Autodesk Inventor part; units mm, degrees
ref_plane "YZ Plane" through (0, 0, 0) normal (1, 0, 0) x (0, 1, 0)
ref_plane "XZ Plane" through (0, 0, 0) normal (0, 1, 0) x (-1, 0, 0)
ref_plane "XY Plane" through (0, 0, 0) normal (0, 0, 1) x (1, 0, 0)
sketch "Sketch1" plane through (0, 0, 0) normal (0, 1, 0) x (-1, 0, 0)
  line L0 (-33.8, -50.05) -> (33.8, -50.05)
  line L1 (33.8, -50.05) -> (33.8, 50.05)
  line L2 (33.8, 50.05) -> (-33.8, 50.05)
  line L3 (-33.8, 50.05) -> (-33.8, -50.05)
  line L4 (-33.8, -50.05) -> (33.8, 50.05) construction
  line L5 (33.8, -50.05) -> (-33.8, 50.05) construction
  point P0 (0, 0)
  dimension "d0" = 67.6
  dimension "d1" = 100.1
extrude "Extrusion1" add sketch "Sketch1" along normal blind 4.445
sketch "Sketch2" plane through (0, 4.445, 0) normal (0, 1, 0) x (1, 0, 0)
  line L0 (30.6, 46.85) -> (-30.6, 46.85)
  line L1 (-30.6, 46.85) -> (-30.6, -46.85)
  line L2 (-30.6, -46.85) -> (30.6, -46.85)
  line L3 (30.6, -46.85) -> (30.6, 46.85)
  line L4 (30.6, 46.85) -> (-30.6, -46.85) construction
  line L5 (-30.6, 46.85) -> (30.6, -46.85) construction
  line L6 (-33.8, 50.05) -> (-33.8, -50.05)
  line L7 (-33.8, -50.05) -> (33.8, -50.05)
  line L8 (33.8, 50.05) -> (-33.8, 50.05)
  line L9 (33.8, -50.05) -> (33.8, 50.05)
  line L10 (27.4, -43.65) -> (33.8, -50.05) construction
  line L11 (24.9431, -46.85) -> (30.9716, -52.8784)
  line L12 (36.6284, -47.2216) -> (30.6, -41.1931)
  arc A0 (30.9716, -52.8784) -> (36.6284, -47.2216) centre (33.8, -50.05) ccw
  circle A1 centre (33.8, -50.05) radius 1.375
  point P0 (0, 0)
  dimension "d4" = 3.2
  dimension "d5" = 3.2
  dimension "d22" = 8
  dimension "d23" = 2.75
extrude "Extrusion2" add sketch "Sketch2" along normal blind 28 contours L0 L1 L2 L11 L7 L6 L8 L9 L12 L3 | L12 L9 A1 L7 L11 L2 L3 | L9 L7 A1 picked at (32.9402, -49.7491)
sketch "Sketch4" plane through (0, 0, 0) normal (0, -1, 0) x (1, 0, 0)
  line L0 (32.2906, 48.7379) -> (35.3094, 51.3621) construction
  line L1 (33.8, 50.05) -> (33.8, -50.05)
  line L2 (33.8, 44.7499) -> (37.9337, 48.3433)
  line L3 (32.6852, 54.381) -> (29.6663, 51.7567)
  arc A0 (29.6663, 51.7567) -> (28.5119, 50.05) centre (32.2906, 48.7379) ccw
  arc A1 (37.9337, 48.3433) -> (32.6852, 54.381) centre (35.3094, 51.3621) ccw
  line L4 (-33.8, 50.05) -> (33.8, 50.05)
  line L5 (28.5119, 50.05) -> (33.8, 50.05)
  line L6 (33.8, 50.05) -> (33.8, 44.7499)
  circle A2 centre (35.3094, 51.3621) radius 1.985
  line L7 (0, 50.05) -> (0, -50.05) construction
  line L8 (33.8, -50.05) -> (-33.8, -50.05) construction
  line L9 (33.8, 0) -> (-33.3, 0) construction
  line L10 (33.8, -50.05) -> (33.8, 50.05)
  line L11 (33.8, -44.7499) -> (37.9337, -48.3433)
  line L12 (32.6852, -54.381) -> (29.6663, -51.7567)
  arc A3 (28.5119, -50.05) -> (29.6663, -51.7567) centre (32.2906, -48.7379) ccw
  arc A4 (32.6852, -54.381) -> (37.9337, -48.3433) centre (35.3094, -51.3621) ccw
  line L13 (-33.8, -50.05) -> (33.8, -50.05)
  circle A5 centre (35.3094, -51.3621) radius 1.985
  line L14 (-33.8, 50.05) -> (-33.8, -50.05)
  line L15 (-33.8, 44.7499) -> (-37.9337, 48.3433)
  line L16 (-32.6852, 54.381) -> (-29.6663, 51.7567)
  arc A6 (-28.5119, 50.05) -> (-29.6663, 51.7567) centre (-32.2906, 48.7379) ccw
  arc A7 (-32.6852, 54.381) -> (-37.9337, 48.3433) centre (-35.3094, 51.3621) ccw
  line L17 (-28.5119, 50.05) -> (-33.8, 50.05)
  circle A8 centre (-35.3094, 51.3621) radius 1.985
  arc A9 (-37.9337, -48.3433) -> (-32.6852, -54.381) centre (-35.3094, -51.3621) ccw
  line L18 (-33.8, -44.7499) -> (-37.9337, -48.3433)
  line L19 (-32.6852, -54.381) -> (-29.6663, -51.7567)
  arc A10 (-29.6663, -51.7567) -> (-28.5119, -50.05) centre (-32.2906, -48.7379) ccw
  circle A11 centre (-35.3094, -51.3621) radius 1.985
  line L20 (-28.5119, -50.05) -> (-33.8, -50.05)
  line L21 (-33.8, -50.05) -> (-33.8, 50.05)
  point P0 (0, 0)
  point P1 (-28.5119, -50.05)
  point P2 (-33.8, -44.7499)
  point P3 (-28.5119, 50.05)
  point P4 (33.8, -44.7499)
  dimension "d24" = 2
  dimension "d25" = 8
  dimension "d26" = 131
  dimension "d27" = 3.97
extrude "Extrusion4" add sketch "Sketch4" against normal up to surface (32.445 mm away) contours L4 A0 L3 A1 L2 L1 | L11 A4 L12 A3 L13 L1 | L4 L14 L15 A7 L16 A6 | A10 L19 A9 L18 L14 L13
fillet "Fillet2" radius 2 4 edges at (30.6, 18.445, -46.85) (-30.6, 18.445, -46.85) (-30.6, 18.445, 46.85) (30.6, 18.445, 46.85)
sketch "Sketch14" plane through (0, 4.445, 0) normal (0, 1, 0) x (1, 0, 0)
  circle A0 centre (27.1, -34.85) radius 3.7
  circle A1 centre (27.1, -34.85) radius 1.985
  line L0 (28.6, -46.85) -> (-28.6, -46.85)
  line L1 (30.6, 44.85) -> (30.6, -44.85)
  line L2 (-28.6, -46.85) -> (28.6, -46.85) construction
  line L3 (0, -46.85) -> (0, 50.05) construction
  line L4 (28.5119, 50.05) -> (-28.5119, 50.05) construction
  circle A2 centre (27.1, 23.15) radius 3.7
  circle A3 centre (27.1, 23.15) radius 1.985
  line L5 (-30.6, 44.85) -> (-30.6, -44.85) construction
  line L6 (-30.6, 0) -> (30.6, 0) construction
  line L7 (30.6, -44.85) -> (30.6, 44.85) construction
  circle A4 centre (-21.9, -34.85) radius 3.7
  circle A5 centre (-21.9, -34.85) radius 1.985
  circle A6 centre (-21.9, 23.15) radius 1.985
  circle A7 centre (-21.9, 23.15) radius 3.7
  point P0 (0, 0)
  dimension "d114" = 7.4
  dimension "d115" = 3.97
  dimension "d116" = 12
  dimension "d117" = 3.5
  dimension "d120" = 58
  dimension "d127" = 49
sketch "Sketch15" plane through (0, 4.445, 0) normal (0, 1, 0) x (1, 0, 0)
  point P0 (0, 0)
extrude "Extrusion10" add sketch "Sketch14" along normal blind 6
sketch "Sketch16" plane through (33.8, 0, 44.7499) normal (1, 0, 0) x (0, 0, -1)
  line L0 (12.9515, 13.2621) -> (12.9515, 13.455)
  line L1 (20.9323, 13.455) -> (20.9323, 13.2621)
  line L2 (13.9419, 14.5004) -> (19.9419, 14.5004)
  line L3 (88.3241, 11.975) -> (9.3999, 11.975)
  line L4 (21.9323, 11.475) -> (11.9515, 11.475)
  line L5 (11.9515, 11.475) -> (11.9515, 15.5004)
  line L6 (11.9515, 15.5004) -> (21.9323, 15.5004)
  line L7 (21.9323, 15.5004) -> (21.9323, 11.475)
  line L8 (30.8419, 17.055) -> (30.8419, 14.5766)
  line L9 (45.8419, 14.5766) -> (45.8419, 17.055)
  line L10 (45.0419, 17.855) -> (31.6419, 17.855)
  line L11 (46.8419, 11.475) -> (29.8419, 11.475)
  line L12 (29.8419, 11.475) -> (29.8419, 18.855)
  line L13 (29.8419, 18.855) -> (46.8419, 18.855)
  line L14 (46.8419, 18.855) -> (46.8419, 11.475)
  line L15 (56.4419, 17.775) -> (56.4419, 11.775)
  line L16 (63.4419, 11.775) -> (63.4419, 17.775)
  line L17 (63.4419, 17.775) -> (59.9419, 17.775)
  line L18 (59.9419, 17.775) -> (56.4419, 17.775)
  line L19 (64.4419, 11.475) -> (55.4419, 11.475)
  line L20 (55.4419, 11.475) -> (55.4419, 18.775)
  line L21 (55.4419, 18.775) -> (64.4419, 18.775)
  line L22 (64.4419, 18.775) -> (64.4419, 11.475)
  point P0 (44.7499, 0)
  dimension "d134" = 1
  dimension "d135" = 0.5
  dimension "d136" = 1
  dimension "d137" = 1
  dimension "d138" = 1
  dimension "d139" = 0.5
  dimension "d140" = 1
  dimension "d141" = 1
  dimension "d142" = 0.5
  dimension "d143" = 1
  dimension "d144" = 1
  dimension "d145" = 1
extrude "Extrusion11" cut sketch "Sketch16" against normal up to surface (3.2 mm away)
sketch "Sketch17" plane through (28.5119, 0, -50.05) normal (0, 0, -1) x (-1, 0, 0)
  line L0 (16.1912, 11.975) -> (16.1912, 25.475)
  line L1 (0.3112, 11.975) -> (0.3112, 25.475)
  line L2 (0.3112, 25.475) -> (16.1912, 25.475)
  line L3 (50.9119, 11.975) -> (0.9119, 11.975)
  line L4 (16.4912, 11.725) -> (0.0112, 11.725)
  line L5 (0.0112, 11.725) -> (0.0112, 25.725)
  line L6 (0.0112, 25.725) -> (16.4912, 25.725)
  line L7 (16.4912, 25.725) -> (16.4912, 11.725)
  line L8 (19.4512, 18.7546) -> (19.4512, 21.7546)
  line L9 (34.5512, 21.7546) -> (34.5512, 18.7546)
  line L10 (24.0012, 27.465) -> (30.0012, 27.465)
  line L11 (35.2512, 11.225) -> (18.7512, 11.225)
  line L12 (18.7512, 11.225) -> (18.7512, 28.465)
  line L13 (18.7512, 28.465) -> (35.2512, 28.465)
  line L14 (35.2512, 28.465) -> (35.2512, 11.225)
  line L15 (37.4512, 18.7546) -> (37.4512, 21.7546)
  line L16 (52.5512, 21.7546) -> (52.5512, 18.7546)
  line L17 (42.0012, 27.465) -> (48.0012, 27.465)
  line L18 (53.2512, 11.225) -> (36.7512, 11.225)
  line L19 (36.7512, 11.225) -> (36.7512, 28.465)
  line L20 (36.7512, 28.465) -> (53.2512, 28.465)
  line L21 (53.2512, 28.465) -> (53.2512, 11.225)
  point P0 (28.5119, 0)
  point P1 (18.7512, 11.975)
  point P2 (35.2512, 11.975)
  dimension "d148" = 0.3
  dimension "d149" = 0.3
  dimension "d150" = 0.25
  dimension "d151" = 0.25
  dimension "d154" = 0.7
  dimension "d155" = 0.7
  dimension "d156" = 1
  dimension "d157" = 0.75
  dimension "d158" = 1
  dimension "d159" = 0.7
  dimension "d160" = 0.7
  dimension "d161" = 0.75
extrude "Extrusion12" cut sketch "Sketch17" against normal up to surface (3.2 mm away)
properties part number "Case Rev D" material "ABS Plastic"
Geometry check sheet. Reference: the model listing, model coordinates, mm. A direction names the side the tool comes from. Coordinates: 2 decimals unless noted, no trailing zeros. Write each loop counter-clockwise with the first axis right and the second up, starting at its lowest first coordinate (ties: lowest second). Pieces come first, ordered by that corner, then holes. Notation, with made-up numbers: M 81,-34.5 L 111,-34.5 A13 ccw 111,-21.5 Z; hole C 7.5,49 d1. An arc over 180 degrees is marked long. One line per item, written item: value. Start each with the question number.
(1) Scan lines: line 1 along Z through (x, y) = (27.1, 8.4) (3 decimals); line 2 along Z through (x, y) = (31.5, 13.5); line 3 along X through (y, z) = (8, -23). Record each from-to range of solid material in increasing order. Write a range as [from, to].
(2) Sectioned sample at A-A, the plane z = -13. Enter the section's corners in (x, y) (3 decimals).
(3) Sectioned sample at B-B, the plane x = 27.1. Enter the section's corners in (y, z) (3 decimals).
(4) Depth check by flat-ended pin: pin 1 (4 mm diameter, centred on y = 10.5, z = -34, fed in from +X); pin 2 (8 mm diameter, centred on x = 19.5, z = 29.5, fed in from +Y) (3 decimals); pin 3 (5 mm diameter, centred on x = 13, z = -28.5, fed in from -Y); pin 4 (14 mm diameter, centred on x = 9, y = 13, fed in from -Z). Enter the tip coordinate at first touch or a pass-through.
(5) Sectioned sample at D-D, the plane y = 20. State how many separate pieces and enclosed holes the cut face has, and give its area (3 significant figures).
(6) Tool access check on faces 1 (the face through (32, 15, -19.692)), 2 (the face through (29, 10.445, 36)), 3 (the face through (-31.2, 16, -53.09)), 4 (the face through (-35.838, 15.995, 46.521)). Record the directions out of +Z, -Z, +X, -X, +Y, -Y that give a thin tool (end or side, any length) a straight path to the whole face; none if there is none.
(7) Release check for a two-part mould opening along X. For faces 5 (the face through (-33.8, 16, -1)), 6 (the face through (-6.739, 20, -48)), 7 (the face through (32, 15.5, 28)), 8 (the face through (38.27, 16, -54.05)) record: released by +X, released by -X, zero draft, split by the parting line, or undercut.
(8) Sectioned sample at C-C, the plane z = 11. Enter the section's corners in (x, y) (3 decimals).
Filled sheet:
1. line 1: [-50.05, -46.85], [-26.85, -25.135], [-21.165, -19.45], [31.15, 32.865], [36.835, 38.55], [46.85, 50.05]
1. line 2: [-53.35, -19.69], [-10.69, -2.09], [14.91, 22.82], [32.8, 53.35]
1. line 3: [-33.8, -30.6], [-25.6, -23.88], [-19.92, -18.2], [23.4, 25.12], [29.08, 33.8]
2. outline: M -33.8,0 L 33.8,0 L 33.8,11.475 L 30.6,11.475 L 30.6,4.445 L -30.6,4.445 L -30.6,32.445 L -33.8,32.445 Z; M 30.6,18.775 L 33.8,18.775 L 33.8,32.445 L 30.6,32.445 Z
3. outline: M 0,-50.05 L 11.725,-50.05 L 11.725,-46.85 L 4.445,-46.85 L 4.445,-26.85 L 10.445,-26.85 L 10.445,-25.135 L 4.445,-25.135 L 4.445,-21.165 L 10.445,-21.165 L 10.445,-19.45 L 4.445,-19.45 L 4.445,31.15 L 10.445,31.15 L 10.445,32.865 L 4.445,32.865 L 4.445,36.835 L 10.445,36.835 L 10.445,38.55 L 4.445,38.55 L 4.445,46.85 L 32.445,46.85 L 32.445,50.05 L 0,50.05 Z; M 25.725,-50.05 L 32.445,-50.05 L 32.445,-46.85 L 25.725,-46.85 Z
4. pin 1: x = 33.8
4. pin 2: y = 4.445
4. pin 3: y = 0
4. pin 4: z = -50.05
5. separate pieces: 3
5. enclosed holes: 4
5. area: 1,060 mm²
6. face 1: +X
6. face 2: +Y
6. face 3: -Z, +Y, -Y
6. face 4: -X, +Y, -Y
7. face 5: released by -X
7. face 6: undercut
7. face 7: zero draft
7. face 8: undercut
8. outline: M -33.8,0 L 33.8,0 L 33.8,11.475 L 30.6,11.475 L 30.6,4.445 L -30.6,4.445 L -30.6,32.445 L -33.8,32.445 Z; M 30.6,18.855 L 33.8,18.855 L 33.8,32.445 L 30.6,32.445 Z
